Model file for the job. Use its own axes, mm. Coordinates: 2 decimals unless noted, no trailing zeros. Write each loop counter-clockwise with the first axis right and the second up, starting at its lowest first coordinate (ties: lowest second). Pieces come first, ordered by that corner, then holes.
Q1. Drill centre lines: probe 1 along Z at (x, y) = (9, -2); probe 2 along Z at (x, y) = (0, -1.4) (3 decimals); probe 3 along X at (y, z) = (-1.5, 7.5). Where is each one in solid material? Low to high.
Q2. Band-saw the part on A-A, the plane x = 0. Write the cut outline in (y, z) (3 decimals).
Q3. Band-saw the part on C-C, the plane z = -9. Write the cut outline in (x, y).
Q4. Pull direction X, two halves, no side cores. Call faces 1 (the cylindrical face through (9.1, -1.5, -13.7)), 2 (the cylindrical face through (0.425, -1.479, 19.345)), 3 (the flat face through (0, -3, -17)): released by +X, released by -X, zero draft, split by the parting line, or undercut.
Q5. Band-saw the part on D-D, the plane x = 8.5. Write the cut outline in (y, z).
Q6. Band-saw the part on B-B, the plane y = -0.75. Write the cut outline in (x, z) (3 decimals).
Q7. Pin check, flat tip, straight feed: P1, Ø3, axis at x = -15, z = 0, coming from the -Y side. Stop position of the tip, or through.
from build123d import *

# Parameters (mm, degrees)
SKETCH_R   = 10.125
SKETCH_R_2 = 1.75
PAD_DEPTH  = 3


with BuildPart() as part:
    # Sketch → Pad (new body)
    with BuildSketch(Plane.XZ):
        with BuildLine():
            ThreePointArc((19.35, -3e-06), (0, 19.35), (-19.35, -3e-06))
            Line((-19.35, -3e-06), (-19.35, -40.000003))
            Line((-19.35, -40.000003), (19.35, -40.000003))
            Line((19.35, -40.000003), (19.35, -3e-06))
        make_face()
        Circle(SKETCH_R, mode=Mode.SUBTRACT)
        with Locations((7.500003, 12.990379)):
            Circle(SKETCH_R_2, mode=Mode.SUBTRACT)
        with Locations((-15, 5e-06)):
            Circle(SKETCH_R_2, mode=Mode.SUBTRACT)
        with Locations((7.499994, -12.990384)):
            Circle(SKETCH_R_2, mode=Mode.SUBTRACT)
    extrude(amount=PAD_DEPTH)


solid = part.part
Answer sheet:
1. probe 1: z = -40 to -13.89, -12.09 to -4.64, 4.64 to 12.09, 13.89 to 17.13
1. probe 2: z = -40 to -10.125, 10.125 to 19.35
1. probe 3: x = -17.84 to -6.8, 6.8 to 17.84
2. outline: (-3, -40) - (0, -40) - (0, -10.125) - (-3, -10.125) - close; (-3, 10.125) - (0, 10.125) - (0, 19.35) - (-3, 19.35) - close
3. outline: (-19.35, -3) - (-4.64, -3) - (-4.64, 0) - (-19.35, 0) - close; (4.64, -3) - (19.35, -3) - (19.35, 0) - (4.64, 0) - close
4. face 1: undercut
4. face 2: split by the parting line
4. face 3: zero draft
5. outline: (-3, -40) - (0, -40) - (0, -14.43) - (-3, -14.43) - close; (-3, -11.55) - (0, -11.55) - (0, -5.5) - (-3, -5.5) - close; (-3, 5.5) - (0, 5.5) - (0, 11.55) - (-3, 11.55) - close; (-3, 14.43) - (0, 14.43) - (0, 17.38) - (-3, 17.38) - close
6. outline: (-19.35, -40) - (19.35, -40) - (19.35, 0) arc R19.35 ccw to (-19.35, 0) - close; hole circle Ø3.5 at (-15, 0); hole circle Ø20.25 at (0, 0); hole circle Ø3.5 at (7.5, -12.99); hole circle Ø3.5 at (7.5, 12.99)
7. P1: passes through
